from build123d import *

# Parameters (mm, degrees)
BOSS_EXTRUDE1_DEPTH    = 127
CUT_EXTRUDE3_OUTLINE_R = 10.16
CUT_EXTRUDE3_DEPTH     = 50.8
CHAMFER3_SIZE          = 5.08
SKETCH2_W              = 19.05
SKETCH2_H              = 76.2
CUT_EXTRUDE4_DEPTH     = 12.7
FILLET2_R              = 12.7
CUT_EXTRUDE10_DEPTH    = 31.75


# Read off the part's stored shape, not the designer's step: Cut-Extrude3
with BuildPart() as part:
    # Sketch1 → Boss-Extrude1 (new body)
    with BuildSketch(Plane.XY):
        Polygon((0, 0), (76.2, 0), (76.2, 19.05), (38.1, 50.8), (0, 50.8), align=None)
    extrude(amount=BOSS_EXTRUDE1_DEPTH)

    # Cut-Extrude3 outline → Cut-Extrude3 (cut)
    with BuildSketch(Plane(origin=(0, 0, 0), x_dir=(1, 0, 0), z_dir=(0, 1, 0))):
        with Locations((19.05, -19.05)):
            Circle(CUT_EXTRUDE3_OUTLINE_R)
    extrude(amount=CUT_EXTRUDE3_DEPTH, mode=Mode.SUBTRACT)

    # Chamfer3
    chamfer3_edges = [part.edges().sort_by_distance(p)[0] for p in [
        (8.89, 50.8, 19.05),
        (8.89, 0, 19.05),
    ]]
    chamfer(chamfer3_edges, length=CHAMFER3_SIZE)

    # Sketch2 → Cut-Extrude4 (cut)
    with BuildSketch(Plane(origin=(0, 50.8, 0), x_dir=(1, 0, 0), z_dir=(0, 1, 0))):
        with Locations((9.525, -88.9)):
            Rectangle(SKETCH2_W, SKETCH2_H)
    extrude(amount=-CUT_EXTRUDE4_DEPTH, mode=Mode.SUBTRACT)

    # Fillet2
    fillet2_edges = [part.edges().sort_by_distance(p)[0] for p in [
        (19.05, 44.45, 50.8),
    ]]
    fillet(fillet2_edges, radius=FILLET2_R)

    # Sketch3 → Cut-Extrude10 (cut)
    with BuildSketch(Plane(origin=(0, 50.8, 0), x_dir=(1, 0, 0), z_dir=(0, 1, 0))):
        with BuildLine():
            Line((76.2, -50.8), (60.198, -50.8))
            ThreePointArc((60.198, -50.8), (47.498, -63.5), (60.198, -76.2))
            Line((60.198, -76.2), (76.2, -76.2))
            Line((76.2, -76.2), (76.2, -50.8))
        make_face()
    extrude(amount=-CUT_EXTRUDE10_DEPTH, mode=Mode.SUBTRACT)


solid = part.part
Input: part model. Units: mm. Frame: model coordinates. A direction names the side the tool comes from. Give positions to 0.01 mm unless a question says otherwise; leave off trailing zeros. Loops run counter-clockwise (first coordinate to the right, second up) from the corner with the lowest first, then second, coordinate; pieces in that order, holes last. Notation, with made-up numbers: M 8.5,82.25 L 41.5,82.25 A32 ccw 41.5,111.25 Z; hole C 28,34 d5. An arc over 180 degrees is marked long. Use CSV: the item, a comma, the result in double quotes.
(1) Pin query (flat end, axial travel): P1, Ø1, axis at y = 43, z = 33.5, coming from the +X side; P2, Ø21, axis at x = 8, z = 104, coming from the +Y side; P3, Ø7.5, axis at x = 63.5, z = 64.5, coming from the +Y side. Return the tip coordinate at first contact, or that it passes through.
Outcome:
P1,"stops at x = 48.06"
P2,"stops at y = 38.1"
P3,"stops at y = 19.05"
(2) Section B-B, the plane z = 78. Return loops of the section in (x, y), plus the area to 3 significant figures.
Outcome:
outline,"M 0,0 L 76.2,0 L 76.2,19.05 L 38.1,50.8 L 19.05,50.8 L 19.05,38.1 L 0,38.1 Z"
area,"3,020 mm²"
(3) Material intervals for L1, parallel to X at y = 18, z = 19.05; L2, parallel to Z at x = 19.05, y = 26.5; L3, parallel to Y at x = 10, z = 67.5, sorted ascending. Write a range as [from, to].
Outcome:
L1,"x = [0, 8.89], [29.21, 76.2]"
L2,"z = [0, 8.89], [29.21, 127]"
L3,"y = [0, 38.1]"
(4) Pull-direction query (X, two-part tool) for faces 4 (the face through (10.735, 46.038, 25.426)), 5 (the face through (0, 26, 63)), 6 (the face through (24, 50.8, 63)); classes: pulls with the +X half, pulls with the -X half, needs draft (parallel to the pull), parting line crosses it, or undercut.
Outcome:
face 4,"undercut"
face 5,"pulls with the -X half"
face 6,"needs draft"
(5) Section A-A, the plane z = 19.05. Return loops of the section in (x, y), plus the area to 3 significant figures.
Outcome:
outline,"M 0,0 L 3.81,0 L 8.89,5.08 L 8.89,45.72 L 3.81,50.8 L 0,50.8 Z; M 29.21,5.08 L 34.29,0 L 76.2,0 L 76.2,19.05 L 38.1,50.8 L 34.29,50.8 L 29.21,45.72 Z"
area,"2,180 mm²"
(6) Section C-C, the plane x = 64.5. Return loops of the section in (y, z), plus the area to 3 significant figures.
Outcome:
outline,"M 0,0 L 28.8,0 L 28.8,50.8 L 19.05,50.8 L 19.05,76.2 L 28.8,76.2 L 28.8,127 L 0,127 Z"
area,"3,410 mm²"
(7) Section D-D, the plane y = 7.5. Return loops of the section in (x, z), plus the area to 3 significant figures.
Outcome:
outline,"M 0,0 L 76.2,0 L 76.2,127 L 0,127 Z; hole C 19.05,19.05 d20.32"
area,"9,350 mm²"
(8) Set-up query: faces 1 (the face through (65, 23, 76.2)), 2 (the face through (15.23, 44.36, 54.42)), 3 (the face through (38, 0, 63)). Return all of +Z, -Z, +X, -X, +Y, -Y with unobstructed straight access to the full face (end or side cutting, diameter ignored); none if empty.
Outcome:
face 1,"+X, +Y"
face 2,"+Z, -X, +Y"
face 3,"+Z, -Z, +X, -X, -Y"
